Geometry: final body of the model. Coordinates: model frame, mm. Face numbers are marked on the shaded views. A direction names the side the tool comes from. Coordinates: 2 decimals unless noted, no trailing zeros. Write each loop counter-clockwise with the first axis right and the second up, starting at its lowest first coordinate (ties: lowest second). Pieces come first, ordered by that corner, then holes. Notation, with made-up numbers: (49.5, 27) - (69.5, 27) arc R30 ccw to (69.5, 64) - close; hole circle Ø5 at (68, 8.25). An arc over 180 degrees is marked (long way). Answer as a JSON object with one key per item and string values. Group by question number.
Item 1: Line query: line 1 along Y through (x, z) = (20, 21); line 2 along Z through (x, y) = (55, 90); line 3 along Z through (x, y) = (15, 7.5). Output: solid intervals per line, ascending. Write a range as from..to.
Item 2: Section C-C on z = 45. Return loops of the section in (x, y), and give its area (3 significant figures).
Item 3: Section A-A on y = 65. Return loops of the section in (x, z).
Item 4: Section B-B on x = 55. Return loops of the section in (y, z).
Item 5: Mould query, pull axis Z, two halves, no side actions, for the marked faces 1, 2, 3 and 4. Classes: pulls with the +Z half, pulls with the -Z half, needs draft (parallel to the pull), parting line crosses it, or undercut.
Item 6: First-contact query: pin 1 Ø16 at (y, z) = (8.5, 42) entering from +X; pin 2 Ø4 at (x, z) = (52.5, 22.5) entering from -Y; pin 3 Ø11.5 at (x, z) = (55, 45) entering from -Y. Flat tips, straight axial feed; report the tip coordinate or a pass-through.
Item 7: Section D-D on z = 31.5. Return loops of the section in (x, y), and give its area (3 significant figures).
Item 8: Set-up query: the marked faces 5, 6 and 7. Return all of +Z, -Z, +X, -X, +Y, -Y with unobstructed straight access to the full face (end or side cutting, diameter ignored); none if empty.
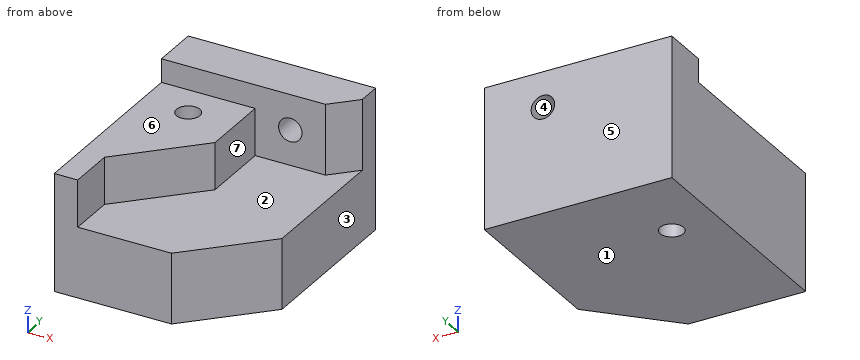
Autodesk Fusion 360 part; units mm, degrees
sketch "Sketch1" plane through (0, 0, 0) normal (0, 0, 1) x (1, 0, 0)
  line L0 (0, 0) -> (50, 0)
  line L1 (0, 0) -> (0, 100)
  line L2 (0, 100) -> (80, 100)
  line L3 (80, 100) -> (80, 90)
  line L4 (80, 90) -> (80, 30)
  line L5 (50, 0) -> (80, 30)
  line L6 (0, 0) -> (10, 0)
  line L7 (10, 0) -> (10, 20)
  line L8 (0, 100) -> (0, 80)
  line L9 (0, 80) -> (70, 80)
  line L10 (70, 80) -> (80, 90)
  line L11 (0, 80) -> (40, 80)
  line L12 (40, 80) -> (40, 50)
  line L13 (10, 20) -> (40, 50)
  circle A0 centre (20, 65) radius 5
extrude "Extrude1" add sketch "Sketch1" along normal blind 50 contours L0 L1 L6 L7 L9 L11 L12 L13
extrude "Extrude2" add sketch "Sketch1" along normal blind 30 contours L0 L4 L5 L7 L9 L10 L12 L13
extrude "Extrude3" add sketch "Sketch1" along normal blind 60 contours L1 L2 L3 L8 L9 L10 L11
sketch "Sketch2" plane through (0, 80, 0) normal (0, -1, 0) x (1, 0, 0)
  line L0 (40, 30) -> (70, 30)
  line L1 (70, 30) -> (70, 60)
  line L2 (70, 60) -> (0, 60)
  line L3 (0, 60) -> (0, 50)
  line L4 (0, 50) -> (40, 50)
  line L5 (40, 50) -> (40, 30)
  circle A0 centre (55, 45) radius 5
extrude "Extrude4" cut sketch "Sketch2" against normal blind 40 contours A0
Checks:
{
 "1": {"line 1": "0..60, 70..100", "line 2": "0..40, 50..60", "line 3": "0..30"},
 "2": {"outline": "(0, 0) - (10, 0) - (10, 20) - (40, 50) - (40, 80) - (50, 80) - (50, 100) - (0, 100) - close; (60, 80) - (70, 80) - (80, 90) - (80, 100) - (60, 100) - close; hole circle Ø10 at (20, 65)", "area": "3,420 mm^2"},
 "3": {"outline": "(0, 0) - (15, 0) - (15, 50) - (0, 50) - close; (25, 0) - (80, 0) - (80, 30) - (40, 30) - (40, 50) - (25, 50) - close"},
 "4": {"outline": "(5, 0) - (100, 0) - (100, 40) - (80, 40) - (80, 30) - (5, 30) - close; (80, 50) - (100, 50) - (100, 60) - (80, 60) - close"},
 "5": {"face 1": "pulls with the -Z half", "face 2": "pulls with the +Z half", "face 3": "needs draft", "face 4": "undercut"},
 "6": {"pin 1": "x = 10", "pin 2": "y = 0.5", "pin 3": "y = 80"},
 "7": {"outline": "(0, 0) - (10, 0) - (10, 20) - (40, 50) - (40, 80) - (70, 80) - (80, 90) - (80, 100) - (0, 100) - close; hole circle Ø10 at (20, 65)", "area": "3,620 mm^2"},
 "8": {"face 5": "+Z, -Z, +X, -X, +Y", "face 6": "+Z, +X, -X, -Y", "face 7": "+Z, +X, -Y"}
}
